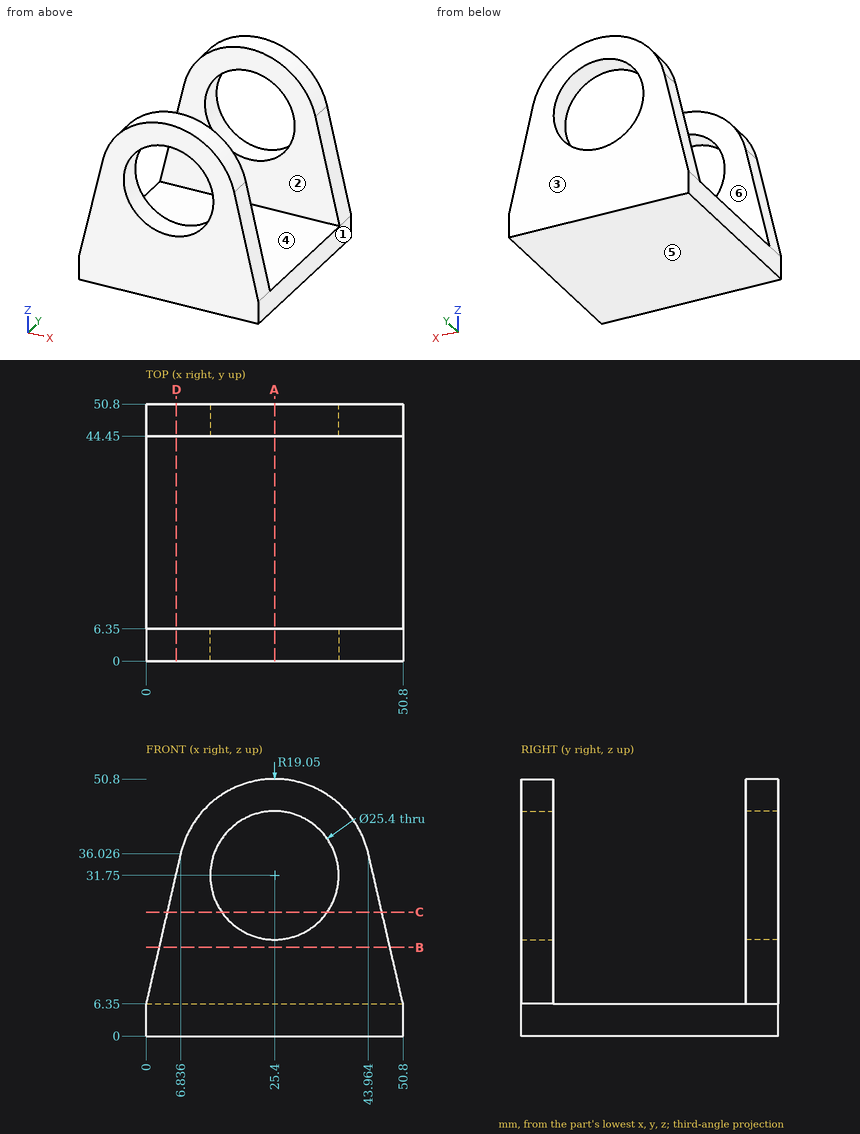
Study the drawing (mm; zero at the part's minimum x, y, z) and answer. A direction names the side the tool comes from. Coordinates: 2 decimals unless noted, no trailing zeros. Loops run counter-clockwise (first coordinate to the right, second up) from the corner with the lowest first, then second, coordinate; pieces in that order, holes last. Notation, with made-up numbers: (-19.5, 86) -> (2.5, 86) arc R14 ccw to (2.5, 96) -> close; hole circle Ø4 at (-5.5, 4.25). An arc over 180 degrees is marked (long way). Answer as CSV lines item,"result".
1) For a pull along Y with two mould halves and no side action, classify the marked faces 1, 2, 3 and 4 as released by +Y, released by -Y, zero draft, split by the parting line, or undercut.
A:
face 1,"zero draft"
face 2,"undercut"
face 3,"released by +Y"
face 4,"undercut"
2) The part is cut by section D-D (x = 6). Give the vertices of the cut face in (y, z).
A:
outline,"(0, 0) -> (50.8, 0) -> (50.8, 32.4) -> (44.45, 32.4) -> (44.45, 6.35) -> (6.35, 6.35) -> (6.35, 32.4) -> (0, 32.4) -> close"
3) Straight lines are drawn through the part: probe 1 along Y at (x, z) = (43, 19.5); probe 2 along Z at (x, y) = (25.4, 48). For each, find the intervals that lie inside material, in ascending order.
A:
probe 1,"y = 0 to 6.35, 44.45 to 50.8"
probe 2,"z = 0 to 19.05, 44.45 to 50.8"
4) The part is cut by section B-B (z = 17.5). Give the vertices of the cut face in (x, y).
A:
outline,"(2.57, 0) -> (48.23, 0) -> (48.23, 6.35) -> (2.57, 6.35) -> close; (2.57, 44.45) -> (48.23, 44.45) -> (48.23, 50.8) -> (2.57, 50.8) -> close"
5) The part is cut by section A-A (x = 25.4). Give the vertices of the cut face in (y, z).
A:
outline,"(0, 0) -> (50.8, 0) -> (50.8, 19.05) -> (44.45, 19.05) -> (44.45, 6.35) -> (6.35, 6.35) -> (6.35, 19.05) -> (0, 19.05) -> close; (0, 44.45) -> (6.35, 44.45) -> (6.35, 50.8) -> (0, 50.8) -> close; (44.45, 44.45) -> (50.8, 44.45) -> (50.8, 50.8) -> (44.45, 50.8) -> close"
6) For the marked faces 5 and 6, determine the directions among +Z, -Z, +X, -X, +Y, -Y from which every point of the face is accessible in a straight line to the end or side of a thin tool.
A:
face 5,"-Z, +X, -X, +Y, -Y"
face 6,"+Z, +X, -X"
7) The part is cut by section C-C (z = 24.5). Give the vertices of the cut face in (x, y), and give its area (3 significant figures).
A:
outline,"(4.18, 0) -> (14.97, 0) -> (14.97, 6.35) -> (4.18, 6.35) -> close; (4.18, 44.45) -> (14.97, 44.45) -> (14.97, 50.8) -> (4.18, 50.8) -> close; (35.83, 0) -> (46.62, 0) -> (46.62, 6.35) -> (35.83, 6.35) -> close; (35.83, 44.45) -> (46.62, 44.45) -> (46.62, 50.8) -> (35.83, 50.8) -> close"
area,"274 mm²"
8) Flat-ended cylindrical pins translate along their axes: pin 1 (5 mm diameter, centred on y = 45.5, z = 37.5, fed in from +X); pin 2 (11.5 mm diameter, centred on x = 13.5, y = 28, fed in from +Z); pin 3 (23 mm diameter, centred on x = 25.4, z = 31.75, fed in from -Y); pin 4 (6 mm diameter, centred on x = 25, y = 40.5, fed in from -Z). Find the tip coordinate at first contact, or state that the pin passes through.
A:
pin 1,"stops at x = 44.2"
pin 2,"stops at z = 6.35"
pin 3,"passes through"
pin 4,"stops at z = 0"
